Source: CAD feature listing. Evaluate the final solid. Frame: model axes, mm. A direction names the side the tool comes from. Coordinates: 2 decimals unless noted, no trailing zeros. Order: outer loops, then holes, each group sorted by start corner. A loop starts at its lowest first (then second) coordinate and runs counter-clockwise, first axis right, second up.
```python
from build123d import *

# Parameters (mm, degrees)
F0_W     = 31.773508
F0_H     = 27.862936
F1_DEPTH = 47.720866
F3_DEPTH = 35.224047
F4_W     = 19.695132
F4_H     = 37.246185
F5_DEPTH = 8.711955


with BuildPart() as f1:
    # F0 (on Top) → F1 (new body)
    with BuildSketch(Plane.XY):
        Rectangle(F0_W, F0_H)
    extrude(amount=F1_DEPTH)

    # F2 (on face) → F3 (cut)
    with BuildSketch(Plane(origin=(-15.886754, 0, 0), x_dir=(0, -1, 0), z_dir=(-1, 0, 0))):
        Polygon((13.931468, 47.720866), (0, 47.720866), (13.931468, 0), align=None)
        Polygon((-13.931468, 11.532108), (-13.931468, 0), (-10.5097, 8.432195), align=None)
    extrude(amount=-F3_DEPTH, mode=Mode.SUBTRACT)

    # F4 (on face) → F5 (cut)
    with BuildSketch(Plane(origin=(0, 13.931468, 0), x_dir=(-1, 0, 0), z_dir=(0, 1, 0))):
        with Locations((0, 30.1552)):
            Rectangle(F4_W, F4_H)
    extrude(amount=-F5_DEPTH, mode=Mode.SUBTRACT)


solid = f1.part
```
Q1. Section query D-D on x = -10.5. Output: boundary loops of the cut face in (y, z), plus the area to 4 significant figures.
Solutions:
outline: (-13.93, 0) - (13.93, 0) - (10.51, 8.43) - (13.93, 11.53) - (13.93, 47.72) - (0, 47.72) - close
area: 977.5 mm2
Q2. Set-up query: faces 4 (the flat face through (-0.222, 12.197, 9.96)), 5 (the flat face through (15.887, 3, 24)), 6 (the flat face through (-9.848, 10, 29)). Return all of +Z, -Z, +X, -X, +Y, -Y with unobstructed straight access to the full face (end or side cutting, diameter ignored); none if empty.
Solutions:
face 4: +X, -X, +Y
face 5: +Z, -Z, +X, +Y, -Y
face 6: +Z, +Y
Q3. Material intervals for line 1 along X through (y, z) = (9.25, 36.5); line 2 along Z through (x, y) = (-5, 11.25); line 3 along Z through (x, y) = (-3, 11.75), sorted ascending.
Solutions:
line 1: x = -15.89 to -9.85, 9.85 to 15.89
line 2: z = 0 to 6.61, 9.1 to 11.53
line 3: z = 0 to 5.38, 9.56 to 11.53
Q4. Section query A-A on x = 5. Output: boundary loops of the cut face in (y, z), plus the area to 3 significant figures.
Solutions:
outline: (-13.93, 0) - (13.93, 0) - (10.51, 8.43) - (13.93, 11.53) - (5.22, 11.53) - (5.22, 47.72) - (0, 47.72) - close
area: 662 mm2
Q5. Section query B-B on y = 8. Output: boundary loops of the cut face in (x, z).
Solutions:
outline: (-15.89, 0) - (15.89, 0) - (15.89, 47.72) - (9.85, 47.72) - (9.85, 11.53) - (-9.85, 11.53) - (-9.85, 47.72) - (-15.89, 47.72) - close
Q6. Pin query (flat end, axial travel): P1, Ø6, axis at x = 0.5, z = 26.5, coming from the +Y side; P2, Ø6, axis at x = 1, z = 31.5, coming from the -Y side; P3, Ø4.5, axis at x = 4.5, y = 8, coming from the +Z side. Return the tip coordinate at first contact, or that it passes through.
Solutions:
P1: stops at y = 5.22
P2: stops at y = -5.61
P3: stops at z = 11.53
Q7. Pull-direction query (Z, two-part tool) for faces 1 (the flat face through (0, 10, 11.532)), 2 (the flat face through (-13, 13.931, 29)), 3 (the flat face through (-0.222, 12.245, 4.157)); classes: pulls with the +Z half, pulls with the -Z half, needs draft (parallel to the pull), parting line crosses it, or undercut.
Solutions:
face 1: pulls with the +Z half
face 2: needs draft
face 3: undercut
Q8. Section query C-C on z = 40.5. Output: boundary loops of the cut face in (x, y).
Solutions:
outline: (-15.89, -2.11) - (15.89, -2.11) - (15.89, 13.93) - (9.85, 13.93) - (9.85, 5.22) - (-9.85, 5.22) - (-9.85, 13.93) - (-15.89, 13.93) - close
